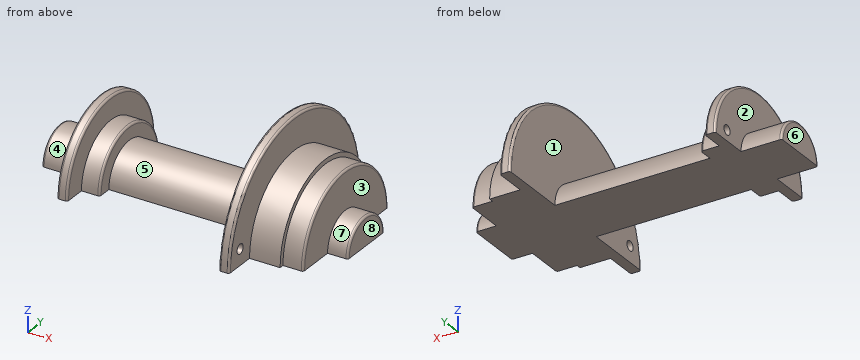
```python
from build123d import *

# Parameters (mm, degrees)
REVOLUTION_ANGLE = 180
SKETCH002_R      = 1.2
POCKET_DEPTH     = 5
SKETCH003_R      = 1.2
POCKET001_DEPTH  = 5
FILLET_R         = 0.5


with BuildPart() as part:
    # Sketch → Revolution (revolve)
    with BuildSketch(Plane.XY):
        Polygon((-37.5, 0), (-37.5, 7), (-27.5, 7), (-27.5, 17), (-25, 17), (-25, 11.5), (-20.5, 11.5), (-20.5, 8), (17.5, 8), (17.5, 25.4), (20, 25.4), (20, 17.5), (27.5, 17.5), (27.5, 16.4), (32.5, 16.4), (32.5, 7), (37.5, 7), (37.5, 0), align=None)
    revolve(axis=Axis((0, 0, 0), (1, 0, 0)), revolution_arc=REVOLUTION_ANGLE)

    # Sketch002 → Pocket (cut)
    with BuildSketch(Plane(origin=(-27.5, 0, 0), x_dir=(0, -1, 0), z_dir=(-1, 0, 0))):
        with Locations((-12.433667, 2.587262)):
            Circle(SKETCH002_R)
    extrude(amount=-POCKET_DEPTH, mode=Mode.SUBTRACT)

    # Sketch003 → Pocket001 (cut)
    with BuildSketch(Plane.YZ.offset(20)):
        with Locations((-21.141078, 3.912139)):
            Circle(SKETCH003_R)
    extrude(amount=-POCKET001_DEPTH, mode=Mode.SUBTRACT)

    # Fillet
    fillet_edges = [part.edges().sort_by_distance(p)[0] for p in [
        (-27.5, 0, 17),
        (-25, 0, 17),
        (-20.5, 0, 11.5),
        (17.5, 0, 25.4),
        (20, 0, 25.4),
        (32.5, 0, 16.4),
        (37.5, 0, 7),
        (-37.5, 0, 7),
    ]]
    fillet(fillet_edges, radius=FILLET_R)


solid = part.part
```
Can you work these out from the model? Positions are in its coordinate system, mm. Face numbers are marked on the shaded views. A direction names the side the tool comes from. Coordinates: 2 decimals unless noted, no trailing zeros. Loops run counter-clockwise (first coordinate to the right, second up) from the corner with the lowest first, then second, coordinate; pieces in that order, holes last. Notation, with made-up numbers: M 76,56.5 L 94,56.5 A8 cw 94,60.5 Z; hole C 4,74 d7. An arc over 180 degrees is marked long. Put each result on its own line as item: value. Start each with the question number.
(1) Imagine slicing it at B-B on x = 5. List the corners of the cut face in (y, z) for me.
(2) Imagine slicing it at C-C on x = 31. List the corners of the cut face in (y, z) for me, and give its area (3 significant figures).
(3) We'd pull the mould along X, two halves only. Please class the marked faces 1, 2 and 3: +X half, -X half, draft (parallel to the pull), parting line (faces both ways), or undercut.
(4) Which directions (+Z, -Z, +X, -X, +Y, -Y) give clear straight access to the entire face, cutting with the end or side of a thin tool? Please do the marked faces 4, 5, 6, 7 and 8.
(5) Imagine slicing it at A-A on y = 0. List the corners of the cut face in (x, z) for me, and give its area (3 significant figures).
(6) Will these pins go through, and if not, where does the flat tip stop? pin 1 Ø10 at (x, y) = (12, -18) entering from +Z; pin 2 Ø5 at (y, z) = (-7.5, 5) entering from -X; pin 3 Ø3 at (y, z) = (12.43, 2.59) entering from +X; pin 4 Ø12 at (x, z) = (5, 3) entering from -Y.
(7) I need wall thicknesses on probe 1 along X at (y, z) = (7.5, 22.5); probe 2 along X at (y, z) = (11, 13.5); probe 3 along Z at (x, y) = (14.5, 7). Which ranges of each line are inside material? Lowest first, please.
Worked answers:
1. outline: M -8,0 L 8,0 A8 ccw Z
2. outline: M -16.4,0 L 16.4,0 A16.4 ccw Z
2. area: 422 mm2
3. face 1: undercut
3. face 2: -X half
3. face 3: +X half
4. face 4: +Z, -X
4. face 5: +Z
4. face 6: +Z, -Z, -X, +Y, -Y
4. face 7: +Z, +X
4. face 8: +Z, -Z, +X, +Y, -Y
5. outline: M -37.5,0 L 37.5,0 L 37.5,6.5 A0.5 ccw 37,7 L 32.5,7 L 32.5,15.9 A0.5 ccw 32,16.4 L 27.5,16.4 L 27.5,17.5 L 20,17.5 L 20,24.9 A0.5 ccw 19.5,25.4 L 18,25.4 A0.5 ccw 17.5,24.9 L 17.5,8 L -20.5,8 L -20.5,11 A0.5 ccw -21,11.5 L -25,11.5 L -25,16.5 A0.5 ccw -25.5,17 L -27,17 A0.5 ccw -27.5,16.5 L -27.5,7 L -37,7 A0.5 ccw -37.5,6.5 Z
5. area: 780 mm2
6. pin 1: passes through
6. pin 2: stops at x = -37.5
6. pin 3: stops at x = 32.5
6. pin 4: stops at y = -8
7. probe 1: x = 17.5 to 20
7. probe 2: x = 17.5 to 27.5
7. probe 3: z = 0 to 3.87
